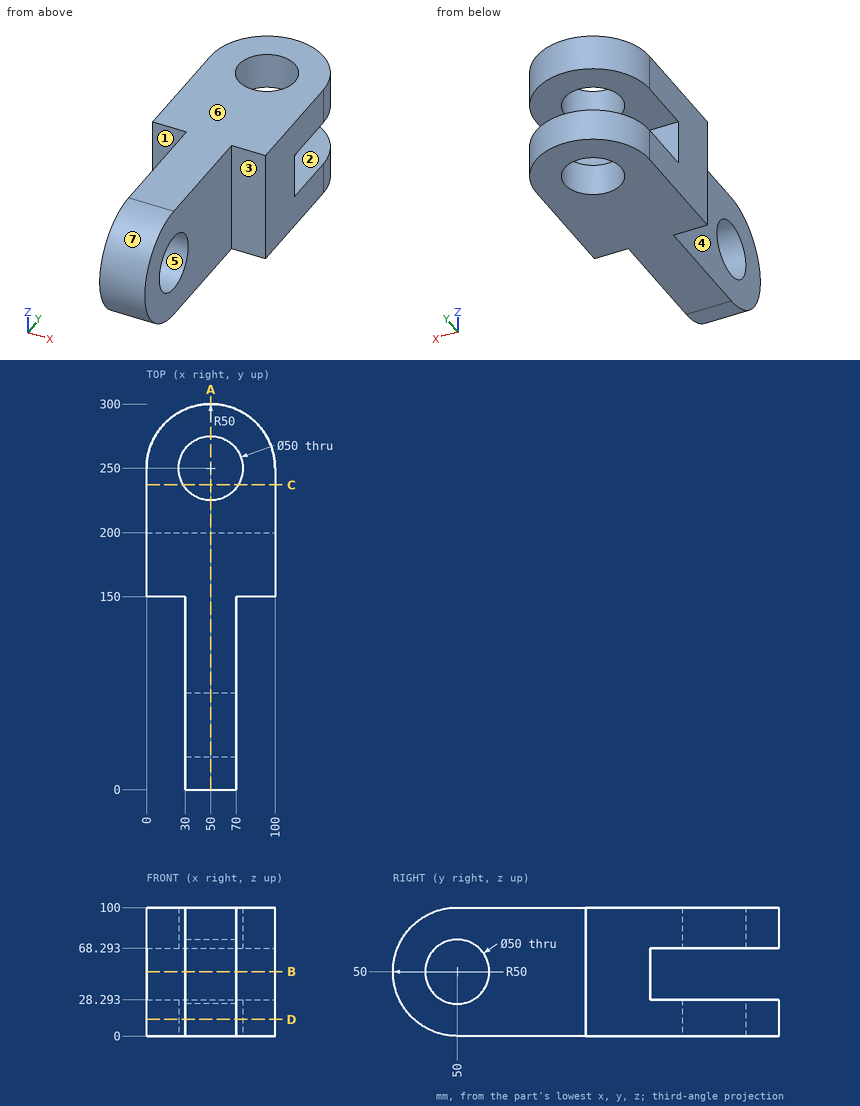
Source: three-view drawing plus pictorial views. Frame: mm from the lowest corner of the part. A direction names the side the tool comes from. Coordinates: 2 decimals unless noted, no trailing zeros. Write each loop counter-clockwise with the first axis right and the second up, starting at its lowest first coordinate (ties: lowest second). Pieces come first, ordered by that corner, then holes. Notation, with made-up numbers: (85, 76.5) -> (98, 76.5) arc R13 ccw to (98, 87.5) -> close; hole circle Ø7 at (-24, -16). An arc over 180 degrees is marked (long way). Answer as a JSON object with one key per item and string values.
1. First-contact query: P1, Ø3, axis at y = 92, z = 47.5, coming from the -X side; P2, Ø24, axis at x = 9.5, z = 27, coming from the -Y side; P3, Ø12, axis at y = 263.5, z = 76, coming from the +X side. Flat tips, straight axial feed; report the tip coordinate or a pass-through.
Result set:
{"P1": "stops at x = 30", "P2": "stops at y = 150", "P3": "stops at x = 99.43"}
2. Section A-A on x = 50. Return the cut outline in (y, z), then the cut area to 3 significant figures.
Result set:
{"outline": "(50, 0) -> (225, 0) -> (225, 28.29) -> (200, 28.29) -> (200, 68.29) -> (225, 68.29) -> (225, 100) -> (50, 100) arc R50 ccw to start; (275, 0) -> (300, 0) -> (300, 28.29) -> (275, 28.29) -> close; (275, 68.29) -> (300, 68.29) -> (300, 100) -> (275, 100) -> close; hole circle Ø50 at (50, 50)", "area": "20,000 mm2"}
3. Section B-B on z = 50. Return the cut outline in (x, y).
Result set:
{"outline": "(0, 150) -> (30, 150) -> (30, 75) -> (70, 75) -> (70, 150) -> (100, 150) -> (100, 200) -> (0, 200) -> close; (30, 0) -> (70, 0) -> (70, 25) -> (30, 25) -> close"}
4. Section D-D on z = 13. Return the cut outline in (x, y).
Result set:
{"outline": "(0, 150) -> (30, 150) -> (30, 16.37) -> (70, 16.37) -> (70, 150) -> (100, 150) -> (100, 250) arc R50 ccw to (0, 250) -> close; hole circle Ø50 at (50, 250)"}
5. Mould query, pull axis Z, two halves, no side actions, for the marked faces 4, 5, 6 and 7. Classes: released by +Z, released by -Z, zero draft, split by the parting line, or undercut.
Result set:
{"face 4": "zero draft", "face 5": "undercut", "face 6": "released by +Z", "face 7": "split by the parting line"}
6. Material intervals for line 1 (X direction, y = 250, z = 6); line 2 (Z direction, x = 12.5, y = 246.5); line 3 (Y direction, x = 48, z = 77.5), sorted ascending. Write a range as from..to.
Result set:
{"line 1": "x = 0..25, 75..100", "line 2": "z = 0..28.29, 68.29..100", "line 3": "y = 8.24..225.08, 274.92..299.96"}
7. Access query for the marked faces 1, 2 and 3. Directions: +Z, -Z, +X, -X, +Y, -Y. A direction counts if a zero-diameter tool reaches every point of the face in a straight line with its end or side. Return the directions, or none.
Result set:
{"face 1": "+Z, -Z, -X, -Y", "face 2": "+X, -X, +Y", "face 3": "+Z, -Z, +X, -Y"}
8. Section C-C on y = 237. Return the cut outline in (x, z) (1 decimal).
Result set:
{"outline": "(0, 0) -> (28.6, 0) -> (28.6, 28.3) -> (0, 28.3) -> close; (0, 68.3) -> (28.6, 68.3) -> (28.6, 100) -> (0, 100) -> close; (71.4, 0) -> (100, 0) -> (100, 28.3) -> (71.4, 28.3) -> close; (71.4, 68.3) -> (100, 68.3) -> (100, 100) -> (71.4, 100) -> close"}
